Source: CAD feature listing. Evaluate the final solid. Frame: model axes, mm. A direction names the side the tool comes from. Give positions to 0.01 mm unless a question says otherwise; leave off trailing zeros. Loops run counter-clockwise (first coordinate to the right, second up) from the corner with the lowest first, then second, coordinate; pieces in that order, holes last.
from build123d import *

# Parameters (mm, degrees)
DODANIE_WYCI_GNI_CIE1_DEPTH = 40
SZKIC2_R                    = 2
WYTNIJ_WYCI_GNI_CIE1_DEPTH  = 35
SZKIC3_W                    = 38
SZKIC3_H                    = 26
SZKIC3_W_2                  = 20
WYTNIJ_WYCI_GNI_CIE2_DEPTH  = 35
ZAOKR_GLENIE1_R             = 5
SZKIC4_R                    = 1.75
WYTNIJ_WYCI_GNI_CIE3_DEPTH  = 35
WYTNIJ_WYCI_GNI_CIE4_START  = -20.200203
WYTNIJ_WYCI_GNI_CIE4_DEPTH  = 2
WYTNIJ_WYCI_GNI_CIE5_START  = -150
WYTNIJ_WYCI_GNI_CIE5_DEPTH  = 2
SZKIC7_R                    = 2
DODANIE_WYCI_GNI_CIE4_DEPTH = 4
WYTNIJ_WYCI_GNI_CIE6_DEPTH  = 1


with BuildPart() as part:
    # Szkic1 → Dodanie-wyciągnięcie1 (new body)
    with BuildSketch(Plane.XY):
        Polygon((-64.9, -3.1), (-64.9, 5.1), (-69.9, 5.1), (-69.9, -5.1), (-80.1, -5.1), (-80.1, 5.1), (-85.1, 5.1), (-85.1, -10.1), (85.1, -10.1), (85.1, 5.100203132), (80.100203132, 5.100203132), (80.100203132, -5.100203132), (69.899796868, -5.100203132), (69.899796868, 5.100203132), (64.899796868, 5.100203132), (64.899796868, -3.1), align=None)
    extrude(amount=DODANIE_WYCI_GNI_CIE1_DEPTH)

    # Szkic2 → Wytnij-wyciągnięcie1 (cut)
    with BuildSketch(Plane.XZ.offset(10.1)):
        with Locations(Location((-25.5, 33.5, 0), (0, 0, 270))):
            Circle(SZKIC2_R)
        with Locations(Location((-25.5, 6.5, 0), (0, 0, 270))):
            Circle(SZKIC2_R)
        with Locations(Location((25.5, 6.5, 0), (0, 0, 270))):
            Circle(SZKIC2_R)
        with Locations(Location((25.5, 33.5, 0), (0, 0, 270))):
            Circle(SZKIC2_R)
    extrude(amount=-WYTNIJ_WYCI_GNI_CIE1_DEPTH, mode=Mode.SUBTRACT)

    # Szkic3 → Wytnij-wyciągnięcie2 (cut)
    with BuildSketch(Plane.XZ.offset(10.1)):
        with Locations((0, 20)):
            Rectangle(SZKIC3_W, SZKIC3_H)
        with Locations((-43, 20)):
            Rectangle(SZKIC3_W_2, SZKIC3_H)
        with Locations((43, 20)):
            Rectangle(SZKIC3_W_2, SZKIC3_H)
    extrude(amount=-WYTNIJ_WYCI_GNI_CIE2_DEPTH, mode=Mode.SUBTRACT)

    # Zaokrąglenie1
    zaokr_glenie1_edges = [part.edges().sort_by_distance(p)[0] for p in [
        (19, -6.6, 33),
        (19, -6.6, 7),
        (-19, -6.6, 7),
        (-19, -6.6, 33),
        (53, -6.6, 33),
        (53, -6.6, 7),
        (33, -6.6, 7),
        (33, -6.6, 33),
        (-33, -6.6, 33),
        (-33, -6.6, 7),
        (-53, -6.6, 7),
        (-53, -6.6, 33),
    ]]
    fillet(zaokr_glenie1_edges, radius=ZAOKR_GLENIE1_R)

    # Szkic4 → Wytnij-wyciągnięcie3 (cut)
    with BuildSketch(Plane(origin=(85.1, 0, 0), x_dir=(0, 0, -1), z_dir=(1, 0, 0))):
        with Locations((-31, 0.100203132)):
            Circle(SZKIC4_R)
        with Locations((-9, 0.100203132)):
            Circle(SZKIC4_R)
    wytnij_wyci_gni_cie3 = extrude(amount=-WYTNIJ_WYCI_GNI_CIE3_DEPTH, mode=Mode.SUBTRACT)

    # Szkic5 → Wytnij-wyciągnięcie4 (cut)
    with BuildSketch(Plane(origin=(85.1, 0, 0), x_dir=(0, 0, -1), z_dir=(1, 0, 0)).offset(WYTNIJ_WYCI_GNI_CIE4_START)):
        Polygon((-29.267949192, 3.100203132), (-32.732050808, 3.100203132), (-34.464101615, 0.100203132), (-32.732050808, -2.899796868), (-29.267949192, -2.899796868), (-27.535898385, 0.100203132), align=None)
        Polygon((-7.267949192, 3.100203132), (-10.732050808, 3.100203132), (-12.464101615, 0.100203132), (-10.732050808, -2.899796868), (-7.267949192, -2.899796868), (-5.535898385, 0.100203132), align=None)
    extrude(amount=WYTNIJ_WYCI_GNI_CIE4_DEPTH, mode=Mode.SUBTRACT)

    # Lustro1: Wytnij-wyciągnięcie3 across plane
    add(wytnij_wyci_gni_cie3.mirror(Plane(origin=(0, 0, 0), x_dir=(0, 0, 1), z_dir=(1, 0, 0))), mode=Mode.SUBTRACT)

    # Szkic5<2> → Wytnij-wyciągnięcie5 (cut)
    with BuildSketch(Plane(origin=(85.1, 0, 0), x_dir=(0, 0, -1), z_dir=(1, 0, 0)).offset(WYTNIJ_WYCI_GNI_CIE5_START)):
        Polygon((-29.267949192, 3.100203132), (-32.732050808, 3.100203132), (-34.464101615, 0.100203132), (-32.732050808, -2.899796868), (-29.267949192, -2.899796868), (-27.535898385, 0.100203132), align=None)
        Polygon((-7.267949192, 3.100203132), (-10.732050808, 3.100203132), (-12.464101615, 0.100203132), (-10.732050808, -2.899796868), (-7.267949192, -2.899796868), (-5.535898385, 0.100203132), align=None)
    extrude(amount=-WYTNIJ_WYCI_GNI_CIE5_DEPTH, mode=Mode.SUBTRACT)

    # Szkic7 → Dodanie-wyciągnięcie4 (add)
    # profile 1 of 2: a face of its own
    with BuildSketch(Plane.XY.offset(40)):
        with BuildLine():
            Line((35, -0.1), (35, -3.1))
            Line((35, -3.1), (45, -3.1))
            Line((45, -3.1), (45, -0.1))
            ThreePointArc((45, -0.1), (40, 4.9), (35, -0.1))
        make_face()
        with Locations((40, -0.1)):
            Circle(SZKIC7_R, mode=Mode.SUBTRACT)
    # profile 2 of 2: a face of its own
    with BuildSketch(Plane.XY.offset(40)):
        with BuildLine():
            ThreePointArc((-35, -0.1), (-40, 4.9), (-45, -0.1))
            Line((-45, -0.1), (-45, -3.1))
            Line((-45, -3.1), (-35, -3.1))
            Line((-35, -3.1), (-35, -0.1))
        make_face()
        with Locations((-40, -0.1)):
            Circle(SZKIC7_R, mode=Mode.SUBTRACT)
    dodanie_wyci_gni_cie4 = extrude(amount=-DODANIE_WYCI_GNI_CIE4_DEPTH)

    # Szkic8 → Wytnij-wyciągnięcie6 (cut)
    with BuildSketch(Plane(origin=(0, 0, 36), x_dir=(-1, 0, 0), z_dir=(0, 0, -1))):
        Polygon((-36.535898385, -0.1), (-38.267949192, 2.9), (-41.732050808, 2.9), (-43.464101615, -0.1), (-41.732050808, -3.1), (-38.267949192, -3.1), align=None)
        Polygon((43.464101615, -0.1), (41.732050808, 2.9), (38.267949192, 2.9), (36.535898385, -0.1), (38.267949192, -3.1), (41.732050808, -3.1), align=None)
    wytnij_wyci_gni_cie6 = extrude(amount=-WYTNIJ_WYCI_GNI_CIE6_DEPTH, mode=Mode.SUBTRACT)

    # Lustro3: Dodanie-wyciągnięcie4, Wytnij-wyciągnięcie6 across plane
    add(dodanie_wyci_gni_cie4.mirror(Plane(origin=(0, 0, 20), x_dir=(1, 0, 0), z_dir=(0, 0, -1))))
    add(wytnij_wyci_gni_cie6.mirror(Plane(origin=(0, 0, 20), x_dir=(1, 0, 0), z_dir=(0, 0, -1))), mode=Mode.SUBTRACT)


solid = part.part
1) Cut plane A-A (x = 25.5). Return loops of the section in (y, z).
Checks:
outline: (-10.1, 0) - (-3.1, 0) - (-3.1, 4.5) - (-10.1, 4.5) - close; (-10.1, 8.5) - (-3.1, 8.5) - (-3.1, 31.5) - (-10.1, 31.5) - close; (-10.1, 35.5) - (-3.1, 35.5) - (-3.1, 40) - (-10.1, 40) - close
2) Cut plane B-B (z = 21). Return loops of the section in (x, y), and give its area (3 significant figures).
Checks:
outline: (-85.1, -10.1) - (-53, -10.1) - (-53, -3.1) - (-64.9, -3.1) - (-64.9, 5.1) - (-69.9, 5.1) - (-69.9, -5.1) - (-80.1, -5.1) - (-80.1, 5.1) - (-85.1, 5.1) - close; (-33, -10.1) - (-19, -10.1) - (-19, -3.1) - (-33, -3.1) - close; (19, -10.1) - (33, -10.1) - (33, -3.1) - (19, -3.1) - close; (53, -10.1) - (85.1, -10.1) - (85.1, 5.1) - (80.1, 5.1) - (80.1, -5.1) - (69.9, -5.1) - (69.9, 5.1) - (64.9, 5.1) - (64.9, -3.1) - (53, -3.1) - close
area: 769 mm2
3) Ray query, probe 1 along X at (y, z) = (-1.25, 17.5); probe 2 along X at (y, z) = (-4.75, 6.5); probe 3 along X at (y, z) = (-4.75, 27). Return the intervals inside material, ascending.
Checks:
probe 1: x = -85.1 to -80.1, -69.9 to -64.9, 64.9 to 69.9, 80.1 to 85.1
probe 2: x = -85.1 to -80.1, -69.9 to -27.5, -23.5 to 23.5, 27.5 to 69.9, 80.1 to 85.1
probe 3: x = -85.1 to -80.1, -69.9 to -53, -33 to -19, 19 to 33, 53 to 69.9, 80.1 to 85.1
4) Contact query for flat-ended pins moving along their axis: P1, Ø1.8, axis at y = 0, z = 31.5, coming from the +X side; P2, Ø4, axis at x = -2.5, z = 31.5, coming from the +Y side. Output: stop coordinate, or through.
Checks:
P1: passes through
P2: stops at y = -3.1
5) Pull-direction query (Z, two-part tool) for faces 4 (the flat face through (45, -2, 38)), 5 (the flat face through (19, -7, 20)); classes: released by +Z, released by -Z, zero draft, split by the parting line, or undercut.
Checks:
face 4: zero draft
face 5: undercut
6) Reachability of faces 1 (the flat face through (39, 2, 37)), 2 (the flat face through (0, -7, 7)), 3 (the cylindrical face through (38.002, -0.012, 38.521)) from +Z, -Z, +X, -X, +Y, -Y: full face, straight path, thin tool, end or side. Return the list, or none.
Checks:
face 1: none
face 2: +Y, -Y
face 3: +Z, -Z
